Geometry check sheet. Reference: the model listing, model coordinates, mm. A direction names the side the tool comes from. Round coordinates to 2 decimals unless told otherwise and drop trailing zeros. Order: outer loops, then holes, each group sorted by start corner. A loop starts at its lowest first (then second) coordinate and runs counter-clockwise, first axis right, second up.
(1) Material ranges on line 1 along Y through (x, z) = (3, 15); line 2 along Y through (x, z) = (-5, -4.5), recorded low to high.
(2) Sectioned sample at A-A (z = 0). Record the boundary of the cut face in (x, y), plus the area to 3 significant figures.
(3) Go/stop test with flat-tipped pins: pin 1 (2 mm diameter, centred on x = -4, y = 35, fed in from +Z); pin 2 (3 mm diameter, centred on x = 9.5, z = -12, fed in from -Y); pin 3 (6 mm diameter, centred on x = 16.5, z = 10.5, fed in from +Y); pin 4 (4 mm diameter, centred on x = 5.5, y = 35.5, fed in from -Z). Record where each tip stops, or that it passes through.
(4) Sectioned sample at C-C (y = 50.5). Record the boundary of the cut face in (x, z), plus the area to 3 significant figures.
(5) Sectioned sample at B-B (x = 0). Record the boundary of the cut face in (y, z).
(6) Set-up check for faces 1 (the face through (-10.74, 33.99, -2.38)), 2 (the face through (0, 16, 21)): record each of +Z, -Z, +X, -X, +Y, -Y from which the full face is reachable in a straight line by a thin tool's end or side.
(7) Sectioned sample at D-D (z = -5). Record the boundary of the cut face in (x, y), plus the area to 3 significant figures.
from build123d import *

# Parameters (mm, degrees)
SKETCH1_W           = 42
SKETCH1_H           = 42
BOSS_EXTRUDE1_DEPTH = 33
SKETCH2_R           = 11
BOSS_EXTRUDE2_DEPTH = 2
SKETCH3_R           = 2.5
BOSS_EXTRUDE3_DEPTH = 22


with BuildPart() as part:
    # Sketch1 → Boss-Extrude1 (new body)
    with BuildSketch(Plane(origin=(0, 0, 0), x_dir=(1, 0, 0), z_dir=(0, 1, 0))):
        Rectangle(SKETCH1_W, SKETCH1_H)
    extrude(amount=BOSS_EXTRUDE1_DEPTH)

    # Sketch2 → Boss-Extrude2 (add)
    with BuildSketch(Plane(origin=(0, 33, 0), x_dir=(1, 0, 0), z_dir=(0, 1, 0))):
        with Locations(Location((0, 0, 0), (0, 0, 270))):
            Circle(SKETCH2_R)
    extrude(amount=BOSS_EXTRUDE2_DEPTH)

    # Sketch3 → Boss-Extrude3 (add)
    with BuildSketch(Plane(origin=(0, 35, 0), x_dir=(1, 0, 0), z_dir=(0, 1, 0))):
        with Locations(Location((0, 0, 0), (0, 0, 270))):
            Circle(SKETCH3_R)
    extrude(amount=BOSS_EXTRUDE3_DEPTH)


solid = part.part
Answer below:
1. line 1: y = 0 to 33
1. line 2: y = 0 to 35
2. outline: (-21, 0) - (21, 0) - (21, 33) - (11, 33) - (11, 35) - (2.5, 35) - (2.5, 57) - (-2.5, 57) - (-2.5, 35) - (-11, 35) - (-11, 33) - (-21, 33) - close
2. area: 1,540 mm2
3. pin 1: stops at z = 10.58
3. pin 2: stops at y = 0
3. pin 3: stops at y = 33
3. pin 4: stops at z = -10.41
4. outline: circle Ø5 at (0, 0)
4. area: 19.6 mm2
5. outline: (0, -21) - (33, -21) - (33, -11) - (35, -11) - (35, -2.5) - (57, -2.5) - (57, 2.5) - (35, 2.5) - (35, 11) - (33, 11) - (33, 21) - (0, 21) - close
6. face 1: +Y
6. face 2: +Z, +X, -X, +Y, -Y
7. outline: (-21, 0) - (21, 0) - (21, 33) - (9.8, 33) - (9.8, 35) - (-9.8, 35) - (-9.8, 33) - (-21, 33) - close
7. area: 1,430 mm2
